```python
from build123d import *

# Parameters (mm, degrees)
SKETCH1_R           = 1.5
BOSS_EXTRUDE1_DEPTH = 2
FILLET4_R           = 20
FILLET5_R           = 10


with BuildPart() as part:
    # Sketch1 → Boss-Extrude1 (new body)
    with BuildSketch(Plane(origin=(0, 0, 0), x_dir=(1, 0, 0), z_dir=(0, 1, 0))):
        Polygon((-17.984046201, 0), (332.015953799, 0), (232.015953799, 84), (32.015953799, 84), align=None)
        with Locations((42.015953799, 20)):
            Circle(SKETCH1_R, mode=Mode.SUBTRACT)
        with Locations((62.015953799, 20)):
            Circle(SKETCH1_R, mode=Mode.SUBTRACT)
        with Locations((82.015953799, 20)):
            Circle(SKETCH1_R, mode=Mode.SUBTRACT)
        with Locations((102.015953799, 20)):
            Circle(SKETCH1_R, mode=Mode.SUBTRACT)
        with Locations((122.015953799, 20)):
            Circle(SKETCH1_R, mode=Mode.SUBTRACT)
        with Locations((22.015953799, 20)):
            Circle(SKETCH1_R, mode=Mode.SUBTRACT)
        with Locations((162.015953799, 20)):
            Circle(SKETCH1_R, mode=Mode.SUBTRACT)
        with Locations((182.015953799, 20)):
            Circle(SKETCH1_R, mode=Mode.SUBTRACT)
        with Locations((202.015953799, 20)):
            Circle(SKETCH1_R, mode=Mode.SUBTRACT)
        with Locations((222.015953799, 20)):
            Circle(SKETCH1_R, mode=Mode.SUBTRACT)
        with Locations((242.015953799, 20)):
            Circle(SKETCH1_R, mode=Mode.SUBTRACT)
        with Locations((142.015953799, 20)):
            Circle(SKETCH1_R, mode=Mode.SUBTRACT)
        with Locations((242.015953799, 60)):
            Circle(SKETCH1_R, mode=Mode.SUBTRACT)
        with Locations((222.015953799, 60)):
            Circle(SKETCH1_R, mode=Mode.SUBTRACT)
        with Locations((202.015953799, 60)):
            Circle(SKETCH1_R, mode=Mode.SUBTRACT)
        with Locations((182.015953799, 60)):
            Circle(SKETCH1_R, mode=Mode.SUBTRACT)
        with Locations((162.015953799, 60)):
            Circle(SKETCH1_R, mode=Mode.SUBTRACT)
        with Locations((142.015953799, 60)):
            Circle(SKETCH1_R, mode=Mode.SUBTRACT)
        with Locations((122.015953799, 60)):
            Circle(SKETCH1_R, mode=Mode.SUBTRACT)
        with Locations((102.015953799, 60)):
            Circle(SKETCH1_R, mode=Mode.SUBTRACT)
        with Locations((82.015953799, 60)):
            Circle(SKETCH1_R, mode=Mode.SUBTRACT)
        with Locations((62.015953799, 60)):
            Circle(SKETCH1_R, mode=Mode.SUBTRACT)
        with Locations((42.015953799, 60)):
            Circle(SKETCH1_R, mode=Mode.SUBTRACT)
        with Locations((282.015953799, 20)):
            Circle(SKETCH1_R, mode=Mode.SUBTRACT)
        with Locations((262.015953799, 20)):
            Circle(SKETCH1_R, mode=Mode.SUBTRACT)
        with Locations((262.015953799, 40)):
            Circle(SKETCH1_R, mode=Mode.SUBTRACT)
        with Locations((242.015953799, 40)):
            Circle(SKETCH1_R, mode=Mode.SUBTRACT)
        with Locations((202.015953799, 40)):
            Circle(SKETCH1_R, mode=Mode.SUBTRACT)
        with Locations((182.015953799, 40)):
            Circle(SKETCH1_R, mode=Mode.SUBTRACT)
        with Locations((162.015953799, 40)):
            Circle(SKETCH1_R, mode=Mode.SUBTRACT)
        with Locations((142.015953799, 40)):
            Circle(SKETCH1_R, mode=Mode.SUBTRACT)
        with Locations((122.015953799, 40)):
            Circle(SKETCH1_R, mode=Mode.SUBTRACT)
        with Locations((102.015953799, 40)):
            Circle(SKETCH1_R, mode=Mode.SUBTRACT)
        with Locations((82.015953799, 40)):
            Circle(SKETCH1_R, mode=Mode.SUBTRACT)
        with Locations((62.015953799, 40)):
            Circle(SKETCH1_R, mode=Mode.SUBTRACT)
        with Locations((42.015953799, 40)):
            Circle(SKETCH1_R, mode=Mode.SUBTRACT)
        with Locations((22.015953799, 40)):
            Circle(SKETCH1_R, mode=Mode.SUBTRACT)
        with Locations((222.015953799, 40)):
            Circle(SKETCH1_R, mode=Mode.SUBTRACT)
        with Locations((32.015953799, 50.397368307)):
            Circle(SKETCH1_R, mode=Mode.SUBTRACT)
    extrude(amount=BOSS_EXTRUDE1_DEPTH)

    # Fillet4
    fillet4_edges = [part.edges().sort_by_distance(p)[0] for p in [
        (332.015953799, 1, 0),
    ]]
    fillet(fillet4_edges, radius=FILLET4_R)

    # Fillet5
    fillet5_edges = [part.edges().sort_by_distance(p)[0] for p in [
        (-17.984046201, 1, 0),
    ]]
    fillet(fillet5_edges, radius=FILLET5_R)


solid = part.part
```
For this review, take the finished solid that the model builds, in its own axes (mm). Coordinates: 2 decimals unless noted, no trailing zeros. Loops run counter-clockwise (first coordinate to the right, second up) from the corner with the lowest first, then second, coordinate; pieces in that order, holes last.
1. Insertion check: P1, Ø1, axis at y = 2, z = -25.5, coming from the -X side. The pin has a flat end and moves straight along its axis. Give the tip position at first contact, or say it passes through.
2. Add section C-C, the plane z = -27. Give the boundary of the cut face in (x, y), then the cut area to 3 significant figures.
3. For line 1 (Z direction, x = 122, y = 0.9); line 2 (Z direction, x = 201, y = 1.55); line 3 (X direction, y = 1.8, z = -16), list the stretches that pass through material, from the lowest coordinate up.
4. Add section B-B, the plane z = -66. Give the boundary of the cut face in (x, y), then the cut area to 3 significant figures.
5. Add section A-A, the plane y = 1.65. Count the separate pieces of the cut face and the enclosed holes in it, then the cut area to 3 significant figures.
Result:
1. P1: stops at x = -3.1
2. outline: (-1.91, 0) - (295.85, 0) - (295.85, 2) - (-1.91, 2) - close
2. area: 596 mm2
3. line 1: z = -84 to -61.5, -58.5 to -41.5, -38.5 to -21.5, -18.5 to 0
3. line 2: z = -84 to -61.1, -58.9 to -41.1, -38.9 to -21.1, -18.9 to 0
3. line 3: x = -8.46 to 296.71
4. outline: (21.3, 0) - (253.44, 0) - (253.44, 2) - (21.3, 2) - close
4. area: 464 mm2
5. separate pieces: 1
5. enclosed holes: 39
5. area: 22,100 mm2
